Here's how the part is built. I have some questions about the finished solid (model axes, mm). A direction names the side the tool comes from. Give positions to 0.01 mm unless a question says otherwise; leave off trailing zeros. Order: outer loops, then holes, each group sorted by start corner. A loop starts at its lowest first (then second) coordinate and runs counter-clockwise, first axis right, second up. Notation, with made-up numbers: M -23,-17.75 L -10,-17.75 A6 ccw -10,-6.75 Z; hole C 20,39 d2. An arc over 180 degrees is marked long. Use one line per item in the form item = value.
from build123d import *

# Parameters (mm, degrees)
F0_W      = 107.442
F0_H      = 22.86
F1_DEPTH  = 8.763
F2_W      = 44.958
F2_H      = 6.7985991507
F3_DEPTH  = 25.4
F4_W      = 44.958
F4_H      = 17.145
F5_DEPTH  = 3.302
F6_W      = 44.958
F6_H      = 17.145
F7_DEPTH  = 3.302
F8_R      = 2.1717
F8_R_2    = 3.81
F9_DEPTH  = 2.54
F10_R     = 4.064
F11_DEPTH = 3.175
F12_R     = 2.54
F14_DEPTH = 6.35
F16_DEPTH = 4.445


with BuildPart() as f1:
    # F0 (on Front) → F1 (new body)
    with BuildSketch(Plane.XZ):
        Rectangle(F0_W, F0_H)
    extrude(amount=F1_DEPTH)

    # F2 (on face) → F3 (cut)
    with BuildSketch(Plane.XZ.offset(8.763)):
        with Locations((0, 10.8926433936)):
            Rectangle(F2_W, F2_H)
        with Locations((0, -13.0509557571)):
            Rectangle(F2_W, F2_H)
    extrude(amount=-F3_DEPTH, mode=Mode.SUBTRACT)

    # F4 (on face) → F5 (cut)
    with BuildSketch(Plane.XZ.offset(8.763)):
        with Locations((0, -1.0791561817)):
            Rectangle(F4_W, F4_H)
    extrude(amount=-F5_DEPTH, mode=Mode.SUBTRACT)

    # F6 (on face) → F7 (cut)
    with BuildSketch(Plane(origin=(0, 0, 0), x_dir=(-1, 0, 0), z_dir=(0, 1, 0))):
        with Locations((0, -1.0791561817)):
            Rectangle(F6_W, F6_H)
    extrude(amount=-F7_DEPTH, mode=Mode.SUBTRACT)

    # F8 (on face) → F9 (join)
    with BuildSketch(Plane.XZ.offset(8.763)):
        with Locations((-26.162, 0)):
            Circle(F8_R)
        with Locations((26.162, 0)):
            Circle(F8_R)
        with Locations((42.164, 0)):
            Circle(F8_R_2)
        with Locations((-42.164, 0)):
            Circle(F8_R_2)
    extrude(amount=F9_DEPTH)

    # F10 (on face) → F11 (join)
    with BuildSketch(Plane.XZ.offset(11.303)):
        with Locations((-26.162, 0)):
            Circle(F10_R)
        with Locations((26.162, 0)):
            Circle(F10_R)
    extrude(amount=F11_DEPTH)

    # F12
    f12_edges = [f1.edges().sort_by_distance(p)[0] for p in [
        (-30.226, -14.478, 0),
        (22.098, -14.478, 0),
    ]]
    fillet(f12_edges, radius=F12_R)

    # F13 (on face) → F14 (join)
    with BuildSketch(Plane.XZ.offset(11.303)):
        Polygon((-34.8496852361, 3.0829702859), (-41.1767732048, 7.8758675398), (-48.4910879687, 4.7928972539), (-49.4783147639, -3.0829702859), (-43.1512267952, -7.8758675398), (-35.8369120313, -4.7928972539), align=None)
        Polygon((48.7893377385, 4.3713620418), (41.6909582919, 7.9233918111), (35.0656205534, 3.5520297693), (35.5386622615, -4.3713620418), (42.6370417081, -7.9233918111), (49.2623794466, -3.5520297693), align=None)
    extrude(amount=F14_DEPTH)

    # F15 (on face) → F16 (join)
    with BuildSketch(Plane(origin=(0, 0, 0), x_dir=(-1, 0, 0), z_dir=(0, 1, 0))):
        Polygon((-35.2800293387, 3.1163504593), (-41.4208533342, 7.5198687012), (-48.3048239954, 4.4035182419), (-49.0479706613, -3.1163504593), (-42.9071466658, -7.5198687012), (-36.0231760046, -4.4035182419), align=None)
        Polygon((49.2749888468, 2.5562726518), (43.5056973679, 7.4364333133), (36.3947085211, 4.8801606615), (35.0530111532, -2.5562726518), (40.8223026321, -7.4364333133), (47.9332914789, -4.8801606615), align=None)
    extrude(amount=F16_DEPTH)


solid = f1.part
Q1. Thinking about a two-plate mould opening in Y: for faces 1 (the face through (38.358, -10.015, 0.168)), 2 (the face through (45.9, -14.43, -5.77)), 3 (the face through (26, -14.478, 0)), which applies, +Y half, -Y half, draft (parallel to the pull), parting line (faces both ways), or undercut?
Found:
face_1 = undercut
face_2 = draft
face_3 = -Y half
Q2. I want a section at D-D on x = -44.5. Write out the boundary of the cut face in (y, z) (3 decimals), then the cut area to 3 significant figures.
Found:
outline = M -17.653,-6.854 L -11.303,-6.854 L -11.303,-3.01 L -8.763,-3.01 L -8.763,-11.43 L 0,-11.43 L 0,-6.114 L 4.445,-6.114 L 4.445,6.595 L 0,6.595 L 0,11.43 L -8.763,11.43 L -8.763,3.01 L -11.303,3.01 L -11.303,6.475 L -17.653,6.475 Z
area = 357 mm²
Q3. On a 3-axis mill with a long thin cutter (end or side, diameter ignored), from which of +Z, -Z, +X, -X, +Y, -Y can I reach the whole of each face in a straight line? I mean faces 4 (the face through (-37.897, 2.191, -4.962)), 5 (the face through (-30.222, -11.616, 0.179)), 6 (the face through (44, -11.303, 4)). Say none if no direction works.
Found:
face_4 = -Z, +Y
face_5 = -Y
face_6 = none
Q4. I want a section at C-C on x = 37. Write out the boundary of the cut face in (y, z) (3 decimals).
Found:
outline = M -17.653,-5.103 L -11.303,-5.103 L -11.303,4.828 L -17.653,4.828 Z; M -8.763,-11.43 L 0,-11.43 L 0,-4.846 L 4.445,-4.846 L 4.445,4.35 L 0,4.35 L 0,11.43 L -8.763,11.43 Z
Q5. I'm going to push flat-ended pins straight in: pin 1 Ø5 at (x, z) = (8.5, 2) entering from -Y; pin 2 Ø13.5 at (x, z) = (-0.5, -0.5) entering from +Y; pin 3 Ø0.6 at (x, y) = (-6.5, -4) entering from +Z; pin 4 Ø12 at (x, y) = (9, -14.5) entering from -Z. Where does each tip first touch, or does it pass through?
Found:
pin_1 = -5.46
pin_2 = -3.3
pin_3 = 7.49
pin_4 = through
Q6. I want a section at B-B on y = 1.75. Write out the boundary of the cut face in (x, z).
Found:
outline = M -49.27,2.56 L -47.93,-4.88 L -40.82,-7.44 L -35.05,-2.56 L -36.39,4.88 L -43.51,7.44 Z; M 35.28,3.12 L 36.02,-4.4 L 42.91,-7.52 L 49.05,-3.12 L 48.3,4.4 L 41.42,7.52 Z
Q7. I need wall thicknesses on L1, parallel to Z at x = -8, y = -4.5; L2, parallel to Y at x = 31, z = 2; L3, parallel to Y at x = -13, z = -1.75. Which ranges of each line are inside material? Lowest first, please.
Found:
L1 = -9.65 to 7.49
L2 = -8.76 to 0
L3 = -5.46 to -3.3
Q8. I want a section at A-A on z = 9.25. Write out the boundary of the cut face in (x, y), then the cut area to 3 significant figures.
Found:
outline = M -53.72,-8.76 L -22.48,-8.76 L -22.48,0 L -53.72,0 Z; M 22.48,-8.76 L 53.72,-8.76 L 53.72,0 L 22.48,0 Z
area = 548 mm²
